from build123d import *

# Parameters (mm, degrees)
F0_W     = 30.48
F0_H     = 35.56
F0_R     = 1.75
F1_DEPTH = 21.082
F2_R     = 4
F3_DEPTH = 35.56
F4_R     = 6.706248
F5_DEPTH = 5.779999
F6_R     = 6.706248
F7_DEPTH = 5.779999


with BuildPart() as f1:
    # F0 (on Top) → F1 (new body)
    with BuildSketch(Plane.XY):
        with Locations((15.24, -17.78)):
            Rectangle(F0_W, F0_H)
        with Locations((6.35, -29.718)):
            Circle(F0_R, mode=Mode.SUBTRACT)
        with Locations((24.13, -29.718)):
            Circle(F0_R, mode=Mode.SUBTRACT)
        with Locations((6.35, -5.842)):
            Circle(F0_R, mode=Mode.SUBTRACT)
        with Locations((24.13, -5.842)):
            Circle(F0_R, mode=Mode.SUBTRACT)
    extrude(amount=F1_DEPTH)

    # F2 (on face) → F3 (cut, through all)
    with BuildSketch(Plane.XZ.offset(35.56)):
        with Locations((15.24, 10.541)):
            Circle(F2_R)
        with BuildLine():
            ThreePointArc((10.31875, 19.862694), (12.704975, 20.772634), (15.24, 21.082))
            Line((15.24, 21.082), (0, 21.082))
            Line((0, 21.082), (0, 3.175))
            Line((0, 3.175), (2.38125, 5.55625))
            Line((2.38125, 5.55625), (2.38125, 19.862694))
            Line((2.38125, 19.862694), (10.31875, 19.862694))
        make_face()
        with BuildLine():
            ThreePointArc((15.24, 21.082), (17.775025, 20.772634), (20.16125, 19.862694))
            Line((20.16125, 19.862694), (28.09875, 19.862694))
            Line((28.09875, 19.862694), (28.09875, 5.55625))
            Line((28.09875, 5.55625), (30.48, 3.175))
            Line((30.48, 3.175), (30.48, 21.082))
            Line((30.48, 21.082), (15.24, 21.082))
        make_face()
    extrude(amount=-F3_DEPTH, mode=Mode.SUBTRACT)

    # F4 (on face) → F5 (cut)
    with BuildSketch(Plane.XZ.offset(35.56)):
        with Locations((15.24, 10.541)):
            Circle(F4_R)
    extrude(amount=-F5_DEPTH, mode=Mode.SUBTRACT)

    # F6 (on face) → F7 (cut)
    with BuildSketch(Plane(origin=(0, 0, 0), x_dir=(-1, 0, 0), z_dir=(0, 1, 0))):
        with Locations((-15.24, 10.541)):
            Circle(F6_R)
    extrude(amount=-F7_DEPTH, mode=Mode.SUBTRACT)


solid = f1.part
Geometry: final body of the model. Coordinates: model frame, mm. A direction names the side the tool comes from. Give positions to 0.01 mm unless a question says otherwise; leave off trailing zeros. Write each loop counter-clockwise with the first axis right and the second up, starting at its lowest first coordinate (ties: lowest second). Pieces come first, ordered by that corner, then holes.
(1) Mould query, pull axis X, two halves, no side actions, for faces 1 (the flat face through (15, -5.78, 6)), 2 (the flat face through (30.48, -18, 2)), 3 (the flat face through (0, -18, 2)), 4 (the flat face through (6, -18, 19.863)). Classes: released by +X, released by -X, zero draft, split by the parting line, or undercut.
(2) Ray query, line 1 (Y direction, x = 24.13, z = 11); line 2 (X direction, y = -6, z = 16.25); line 3 (Y direction, x = 5, z = 9.5). Return the intervals inside material, ascending.
(3) First-contact query: P1, Ø11.5, axis at y = -19, z = 12, coming from the -X side; P2, Ø2, axis at x = 24.13, y = -5.842, coming from the -Z side; P3, Ø4.5, axis at x = 24.13, y = -29.718, coming from the -Z side; P4, Ø3, axis at x = 5.5, y = -32, coming from the +Z side. Flat tips, straight axial feed; report the tip coordinate or a pass-through.
(4) Cut plane B-B, the plane y = -28.5. Return loops of the section in (x, z) (3 decimals), then the cut area to 3 significant figures.
(5) Cut plane A-A, the plane x = 24.13. Return loops of the section in (y, z).
(6) Access query for faces 5 (the cylindrical face through (20.56, -2.85, 6.46)), 6 (the flat face through (28.099, -18, 13)), 7 (the flat face through (2.381, -18, 13)), 8 (the cylindrical face through (18.33, -32.71, 4.59)). Directions: +Z, -Z, +X, -X, +Y, -Y. A direction counts if a zero-diameter tool reaches every point of the face in a straight line with its end or side. Return the directions, or none.
(7) Cut plane D-D, the plane x = 14.5. Return loops of the section in (y, z), then the cut area to 3 significant figures.
(8) Cut plane C-C, the plane z = 1.5. Return loops of the section in (x, y), then the cut area to 3 significant figures.
Values follow:
1. face 1: undercut
1. face 2: released by +X
1. face 3: released by -X
1. face 4: zero draft
2. line 1: y = -35.56 to -31.47, -27.97 to -7.59, -4.09 to 0
2. line 2: x = 2.38 to 4.61, 8.09 to 22.39, 25.87 to 28.1
2. line 3: y = -35.56 to -30.83, -28.6 to -6.96, -4.73 to 0
3. P1: stops at x = 2.38
3. P2: passes through
3. P3: stops at z = 0
3. P4: stops at z = 19.86
4. outline: (0, 0) - (5.093, 0) - (5.093, 19.863) - (2.381, 19.863) - (2.381, 5.556) - (0, 3.175) - close; (7.607, 0) - (22.873, 0) - (22.873, 19.863) - (20.161, 19.863) arc R10.541 ccw to (15.24, 21.082) arc R10.541 ccw to (10.319, 19.863) - (7.607, 19.863) - close; (25.387, 0) - (30.48, 0) - (30.48, 3.175) - (28.099, 5.556) - (28.099, 19.863) - (25.387, 19.863) - close; hole circle Ø8 at (15.24, 10.541)
4. area: 390 mm2
5. outline: (-35.56, 0) - (-31.47, 0) - (-31.47, 19.86) - (-35.56, 19.86) - close; (-27.97, 0) - (-7.59, 0) - (-7.59, 19.86) - (-27.97, 19.86) - close; (-4.09, 0) - (0, 0) - (0, 19.86) - (-4.09, 19.86) - close
6. face 5: +Y
6. face 6: +Z, +X, +Y, -Y
6. face 7: +Z, -X, +Y, -Y
6. face 8: -Y
7. outline: (-35.56, 0) - (0, 0) - (0, 3.88) - (-5.78, 3.88) - (-5.78, 6.61) - (-29.78, 6.61) - (-29.78, 3.88) - (-35.56, 3.88) - close; (-35.56, 17.21) - (-29.78, 17.21) - (-29.78, 14.47) - (-5.78, 14.47) - (-5.78, 17.21) - (0, 17.21) - (0, 21.06) - (-35.56, 21.06) - close
7. area: 406 mm2
8. outline: (0, -35.56) - (30.48, -35.56) - (30.48, 0) - (0, 0) - close; hole circle Ø3.5 at (6.35, -29.72); hole circle Ø3.5 at (6.35, -5.84); hole circle Ø3.5 at (24.13, -29.72); hole circle Ø3.5 at (24.13, -5.84)
8. area: 1,050 mm2
